Job drawing, mm, ordinate dimensions from the low corner. One solid piece. Give positions to 0.01 mm unless a question says otherwise; leave off trailing zeros. Order: outer loops, then holes, each group sorted by start corner. A loop starts at its lowest first (then second) coordinate and runs counter-clockwise, first axis right, second up. Notation, with made-up numbers: (13.25, 22) -> (59.25, 22) arc R17 cw to (59.25, 51) -> close; hole circle Ø7 at (62, 22.25). An arc over 180 degrees is marked (long way). Use CSV: the item, a comma, the result in double quotes. Start each with the question number.
1. Cut at B-B on y = 6.35. List the corners of the cut face in (x, z).
2. Cut at A-A on x = 6.35. List the corners of the cut face in (y, z).
3. Drop flat-ended pins along their axis: pin 1 (1.5 mm diameter, centred on y = 10, z = 4, fed in from -X); pin 2 (3 mm diameter, centred on x = 125.4, y = 6.35, fed in from -Z). Give the stop position or say it passes through.
4. Wall check: line 1 (X direction, y = 6.75, z = 2); line 2 (X direction, y = 5.75, z = 0.8); line 3 (X direction, y = 10.75, z = 4.1). Give the ranges that are in metal, low to high. Write a range as from..to.
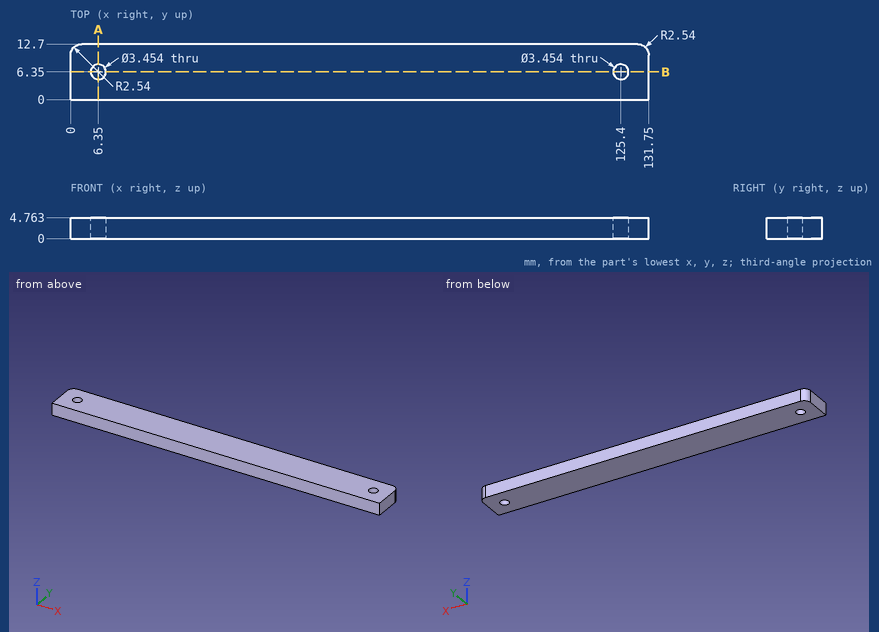
Verdict:
1,outline,"(0, 0) -> (4.62, 0) -> (4.62, 4.76) -> (0, 4.76) -> close; (8.08, 0) -> (123.67, 0) -> (123.67, 4.76) -> (8.08, 4.76) -> close; (127.13, 0) -> (131.75, 0) -> (131.75, 4.76) -> (127.13, 4.76) -> close"
2,outline,"(0, 0) -> (4.62, 0) -> (4.62, 4.76) -> (0, 4.76) -> close; (8.08, 0) -> (12.7, 0) -> (12.7, 4.76) -> (8.08, 4.76) -> close"
3,pin 1,"x = 0"
3,pin 2,"through"
4,line 1,"0..4.67, 8.03..123.72, 127.08..131.75"
4,line 2,"0..4.73, 7.97..123.78, 127.02..131.75"
4,line 3,"0.07..131.68"
